from build123d import *

# Parameters (mm, degrees)
F0_W      = 6.477
F0_H      = 38.1
F0_W_2    = 19.05
F0_H_2    = 5.08
F4_D      = 13.97
F5_W      = 25.4
F5_H      = 25.4
F5_R      = 11.557
F6_DEPTH  = 10.16
F8_DEPTH  = 2.54
F9_R      = 1.984375
F10_DEPTH = 5.08


with BuildPart() as f1:
    # F0 (on Front) → F1 (revolve)
    with BuildSketch(Plane.XZ):
        with Locations((3.2385, 19.05)):
            Rectangle(F0_W, F0_H)
        Polygon((6.477, 38.1), (6.477, 0), (11.557, 0), (11.557, 5.08), (11.557, 22.86), (11.557, 27.94), (11.557, 38.1), align=None)
        with Locations((21.082, 2.54)):
            Rectangle(F0_W_2, F0_H_2)
        with Locations((21.082, 25.4)):
            Rectangle(F0_W_2, F0_H_2)
    revolve(axis=Axis((0, 0, 19.05), (0, 0, 1)))

    # F4 (through all)
    with Locations(Plane.XY.offset(38.1)):
        with Locations((0, 0)):
            Hole(F4_D / 2)

    # F5 (on face) → F6 (join)
    with BuildSketch(Plane.XY.offset(27.94)):
        Rectangle(F5_W, F5_H)
        Circle(F5_R, mode=Mode.SUBTRACT)
    extrude(amount=F6_DEPTH)

    # F7 (on face) → F8 (cut)
    with BuildSketch(Plane.XZ.offset(12.7)):
        Polygon((-1.809819, 29.940453), (1.762056, 29.912878), (3.571875, 32.992424), (1.809819, 36.099547), (-1.762056, 36.127122), (-3.571875, 33.047576), align=None)
    extrude(amount=-F8_DEPTH, mode=Mode.SUBTRACT)

    # F9 (on face) → F10 (cut)
    with BuildSketch(Plane.XZ.offset(10.16)):
        with Locations((0, 33.025466)):
            Circle(F9_R)
    extrude(amount=-F10_DEPTH, mode=Mode.SUBTRACT)


solid = f1.part
Here's how the part is built. I have some questions about the finished solid (model axes, mm). A direction names the side the tool comes from. Coordinates: 2 decimals unless noted, no trailing zeros. Order: outer loops, then holes, each group sorted by start corner. A loop starts at its lowest first (then second) coordinate and runs counter-clockwise, first axis right, second up. Notation, with made-up numbers: M -32.5,37.5 L 22.5,37.5 A20 cw 22.5,74.5 Z; hole C 32.5,-35 d1. An arc over 180 degrees is marked long. Answer as CSV lines item,"result".
Item 1: We'd pull the mould along Z, two halves only. Please class faces 6 (the face through (-12.7, 0, 33)), 7 (the face through (0.4, 7.2, 0)), 8 (the face through (2.703, -11.448, 34.524)): +Z half, -Z half, draft (parallel to the pull), parting line (faces both ways), or undercut.
Results found:
face 6,"draft"
face 7,"-Z half"
face 8,"undercut"
Item 2: Imagine slicing it at D-D on z = 20.5. Write out the boundary of the cut face in (x, y) (3 decimals).
Results found:
outline,"C 0,0 d23.114; hole C 0,0 d13.97"
Item 3: For pin 1 (3 mm diameter, centred on x = 1, z = 34, fed in from -Y); pin 2 (3 mm diameter, centred on x = 5.5, z = 33, fed in from +Y); pin 3 (12 mm diameter, centred on x = -15, z = 30.5, fed in from +Y), each with a flat end and sliding along its axis, tell me the tip position at first contact or that it passes through.
Results found:
pin 1,"y = -10.16"
pin 2,"y = 12.7"
pin 3,"y = 29.07"
Item 4: Imagine slicing it at B-B on x = 27. Write out the boundary of the cut face in (y, z).
Results found:
outline,"M -14.41,0 L 14.41,0 L 14.41,5.08 L -14.41,5.08 Z; M -14.41,22.86 L 14.41,22.86 L 14.41,27.94 L -14.41,27.94 Z"
Item 5: Imagine slicing it at A-A on y = 0. Write out the boundary of the cut face in (x, z) (3 decimals), plus the area to 3 significant figures.
Results found:
outline,"M -30.607,0 L -6.985,0 L -6.985,38.1 L -12.7,38.1 L -12.7,27.94 L -30.607,27.94 L -30.607,22.86 L -11.557,22.86 L -11.557,5.08 L -30.607,5.08 Z; M 6.985,0 L 30.607,0 L 30.607,5.08 L 11.557,5.08 L 11.557,22.86 L 30.607,22.86 L 30.607,27.94 L 12.7,27.94 L 12.7,38.1 L 6.985,38.1 Z"
area,"759 mm2"
Item 6: If I drill on line 1 (Y direction, x = 0, z = 14) (3 decimals); line 2 (Z direction, x = -19, y = 17.5); line 3 (Z direction, x = 0, y = -7.8), over which ranges is the centre line in solid material (lowest first)?
Results found:
line 1,"-11.557 to -6.985, 6.985 to 11.557"
line 2,"0 to 5.08, 22.86 to 27.94"
line 3,"0 to 31.04, 35.01 to 38.1"
Item 7: Imagine slicing it at C-C on x = 0. Write out the boundary of the cut face in (y, z) (3 decimals), plus the area to 3 significant figures.
Results found:
outline,"M -30.607,0 L -6.985,0 L -6.985,31.041 L -10.16,31.041 L -10.16,29.926 L -12.7,29.926 L -12.7,27.94 L -30.607,27.94 L -30.607,22.86 L -11.557,22.86 L -11.557,5.08 L -30.607,5.08 Z; M -12.7,36.114 L -10.16,36.114 L -10.16,35.01 L -6.985,35.01 L -6.985,38.1 L -12.7,38.1 Z; M 6.985,0 L 30.607,0 L 30.607,5.08 L 11.557,5.08 L 11.557,22.86 L 30.607,22.86 L 30.607,27.94 L 12.7,27.94 L 12.7,38.1 L 6.985,38.1 Z"
area,"730 mm2"
Item 8: On a 3-axis mill with a long thin cutter (end or side, diameter ignored), from which of +Z, -Z, +X, -X, +Y, -Y can I reach the whole of each face in a straight line? I mean faces 1 (the face through (2, -10.16, 34)), 2 (the face through (-13, 0, 5.08)), 3 (the face through (-0.2, -12.7, 36.3)), 4 (the face through (5.5, -5.5, 38.1)), 5 (the face through (-24.29, -18.62, 25.44)). Say none if no direction works.
Results found:
face 1,"-Y"
face 2,"none"
face 3,"+Z, +X, -X, -Y"
face 4,"+Z, +X, -X, +Y, -Y"
face 5,"+Z, -Z"
